```python
from build123d import *

# Parameters (mm, degrees)
F0_W          = 165.1
F0_H          = 25.4
F1_DEPTH      = 16.51
F2_R          = 3.81
F3_DEPTH      = 13.97
F5_R          = 2.8575
F6_DEPTH      = 8.382
F6_DEPTH_BACK = 33.782
F7_DEPTH      = 25.4


# Not quite as in the source:
# - a feature names something its author has since deleted; it is built from what else it names


with BuildPart() as f1:
    # F0 (on Front) → F1 (new body)
    with BuildSketch(Plane.XZ):
        with Locations((17.2861106694, 1.5442719363)):
            Rectangle(F0_W, F0_H)
    extrude(amount=F1_DEPTH)

    # F2 (on face) → F3 (join)
    with BuildSketch(Plane.XZ.offset(16.51)):
        with Locations((-57.9527877271, 1.5442719363)):
            Circle(F2_R)
    extrude(amount=F3_DEPTH)

    # F5 (on face) → F6 (join, two sides)
    with BuildSketch(Plane(origin=(0, 0, -11.1557280637), x_dir=(1, 0, 0), z_dir=(0, 0, -1))) as f6_sk:
        with Locations((-46.4608334005, 4.2803706601)):
            Circle(F5_R)
    extrude(amount=F6_DEPTH)
    extrude(f6_sk.sketch, amount=-F6_DEPTH_BACK)

    # F4 (on face) → F7 (join)
    with BuildSketch(Plane(origin=(0, 0, -11.1557280637), x_dir=(1, 0, 0), z_dir=(0, 0, -1))):
        Polygon((99.8361106694, 0), (82.7972726808, 0), (99.8361106694, -15.24), align=None)
    extrude(amount=-F7_DEPTH)


solid = f1.part
```
Work out the finished part from the listing and answer in its coordinate system (mm). A direction names the side the tool comes from. Coordinates: 2 decimals unless noted, no trailing zeros. Loops run counter-clockwise (first coordinate to the right, second up) from the corner with the lowest first, then second, coordinate; pieces in that order, holes last.
1) Section D-D (z = 17.5) is taken. Give the vertices of the cut face in (x, y) (1 decimal).
Results:
outline: circle Ø5.7 at (-46.5, -4.3)
2) Section B-B (x = 1.5) is taken. Give the vertices of the cut face in (y, z), plus the area to 3 significant figures.
Results:
outline: (-16.51, -11.16) - (0, -11.16) - (0, 14.24) - (-16.51, 14.24) - close
area: 419 mm2
3) Section A-A (z = -9) is taken. Give the vertices of the cut face in (x, y).
Results:
outline: (-65.26, -16.51) - (99.84, -16.51) - (99.84, 15.24) - (82.8, 0) - (-65.26, 0) - close
4) Section C-C (y = -28) is taken. Give the vertices of the cut face in (x, z), plus the area to 3 significant figures.
Results:
outline: circle Ø7.62 at (-57.95, 1.54)
area: 45.6 mm2
5) For faces 1 (the flat face through (8, 0, 2)), 2 (the flat face through (-58, -30.48, 2)), 3 (the cylindrical face through (-48.728, -2.542, 18.377)), 4 (the cylindrical face through (-48.728, -2.542, -15.288)), 5 (the cylindrical face through (-61.76, -23.4, 1.71)), determine the directions among +Z, -Z, +X, -X, +Y, -Y from which every point of the face is accessible in a straight line to the end or side of a thin tool.
Results:
face 1: +Z, -Z, -X, +Y
face 2: +Z, -Z, +X, -X, -Y
face 3: +Z
face 4: -Z
face 5: -Y
6) Consider probe 1 along Z at (x, y) = (55.5, -14); probe 2 along Y at (x, z) = (26, -10); probe 3 along Y at (x, z) = (-46.5, -12). Determine where each line is inside the solid, lowest interval first.
Results:
probe 1: z = -11.16 to 14.24
probe 2: y = -16.51 to 0
probe 3: y = -7.14 to -1.42
7) Flat-ended cylindrical pins translate along their axes: pin 1 (12.5 mm diameter, centred on x = 23, z = -3.5, fed in from +Y); pin 2 (1 mm diameter, centred on y = 2.5, z = 10.5, fed in from -X); pin 3 (9.5 mm diameter, centred on x = 54.5, y = -5, fed in from +Z). Find the tip coordinate at first contact, or state that the pin passes through.
Results:
pin 1: stops at y = 0
pin 2: stops at x = 85.03
pin 3: stops at z = 14.24
